Source: CAD feature listing. Evaluate the final solid. Frame: model axes, mm. Face numbers are marked on the shaded views. A direction names the side the tool comes from. Round coordinates to 2 decimals unless told otherwise and drop trailing zeros. Loops run counter-clockwise (first coordinate to the right, second up) from the corner with the lowest first, then second, coordinate; pieces in that order, holes last. Notation, with made-up numbers: M 48.5,-8 L 71.5,-8 A29 cw 71.5,20 Z; hole C 43,19.5 d1. An arc over 180 degrees is marked long. Answer as a JSON object with one key per item and string values.
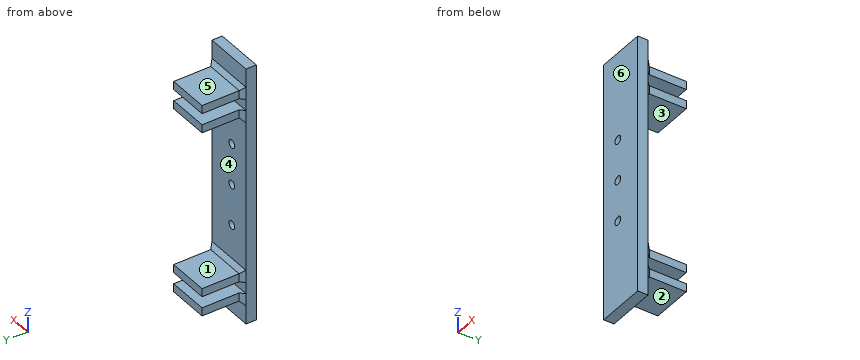
from build123d import *

# Parameters (mm, degrees)
SKETCH1_W               = 24
SKETCH1_H               = 126
BOSS_EXTRUDE1_DEPTH     = 5
SKETCH2_W               = 20
SKETCH2_H               = 4
BOSS_EXTRUDE2_DEPTH     = 20
CUT_EXTRUDE1_DEPTH      = 123.736336331
CUT_EXTRUDE1_DEPTH_BACK = 123.736336331
SKETCH3_R               = 2
CHAMFER1_SIZE           = 2


with BuildPart() as part:
    # Sketch1 → Boss-Extrude1 (new body)
    with BuildSketch(Plane(origin=(0, 0, 0), x_dir=(1, 0, 0), z_dir=(0, 1, 0))):
        with Locations((-62.650887574, -32.349112426)):
            Rectangle(SKETCH1_W, SKETCH1_H)
    extrude(amount=BOSS_EXTRUDE1_DEPTH)

    # Sketch2 → Boss-Extrude2 (add)
    with BuildSketch(Plane(origin=(0, 5, 0), x_dir=(1, 0, 0), z_dir=(0, 1, 0))):
        with Locations((-62.650887574, 17.650887574)):
            Rectangle(SKETCH2_W, SKETCH2_H)
        with Locations((-62.650887574, 8.150887574)):
            Rectangle(SKETCH2_W, SKETCH2_H)
        with Locations((-62.650887574, -72.849112426)):
            Rectangle(SKETCH2_W, SKETCH2_H)
        with Locations((-62.650887574, -82.349112426)):
            Rectangle(SKETCH2_W, SKETCH2_H)
    extrude(amount=BOSS_EXTRUDE2_DEPTH)

    # Sketch3 → Cut-Extrude1 (cut, two sides: drawn at the far end of the back side and taken through both)
    with BuildSketch(Plane(origin=(0, 5, 0), x_dir=(1, 0, 0), z_dir=(0, 1, 0)).offset(-CUT_EXTRUDE1_DEPTH_BACK)):
        with Locations(Location((-64.650887574, -32.349112426, 0), (0, 0, 270))):
            Circle(SKETCH3_R)
        with Locations(Location((-64.650887574, -12.349112426, 0), (0, 0, 270))):
            Circle(SKETCH3_R)
        with Locations(Location((-64.650887574, -52.349112426, 0), (0, 0, 270))):
            Circle(SKETCH3_R)
    extrude(amount=CUT_EXTRUDE1_DEPTH + CUT_EXTRUDE1_DEPTH_BACK, mode=Mode.SUBTRACT)

    # Chamfer1
    chamfer1_edges = [part.edges().sort_by_distance(p)[0] for p in [
        (-72.650887574, 5, -17.650887574),
        (-52.650887574, 5, -17.650887574),
        (-62.650887574, 5, -19.650887574),
        (-72.650887574, 5, -8.150887574),
        (-62.650887574, 5, -6.150887574),
        (-52.650887574, 5, -8.150887574),
        (-72.650887574, 5, 82.349112426),
        (-62.650887574, 5, 84.349112426),
        (-52.650887574, 5, 82.349112426),
        (-62.650887574, 5, 70.849112426),
        (-72.650887574, 5, 72.849112426),
        (-52.650887574, 5, 72.849112426),
    ]]
    chamfer(chamfer1_edges, length=CHAMFER1_SIZE - 0.0001)  # a hair under: the kernel refuses the full size


solid = part.part
Item 1: Access query for the marked faces 1 and 2. Directions: +Z, -Z, +X, -X, +Y, -Y. A direction counts if a zero-diameter tool reaches every point of the face in a straight line with its end or side. Return the directions, or none.
Answer sheet:
{"face 1": "+X, -X, +Y", "face 2": "-Z, +X, -X, +Y"}
Item 2: Section A-A on y = 11.75. Return the cut outline in (x, z), then the cut area to 3 significant figures.
Answer sheet:
{"outline": "M -72.65,-19.65 L -52.65,-19.65 L -52.65,-15.65 L -72.65,-15.65 Z; M -72.65,-10.15 L -52.65,-10.15 L -52.65,-6.15 L -72.65,-6.15 Z; M -72.65,70.85 L -52.65,70.85 L -52.65,74.85 L -72.65,74.85 Z; M -72.65,80.35 L -52.65,80.35 L -52.65,84.35 L -72.65,84.35 Z", "area": "320 mm²"}
Item 3: Section B-B on z = 53. Return the cut outline in (x, y), then the cut area to 3 significant figures.
Answer sheet:
{"outline": "M -74.65,0 L -66.54,0 L -66.54,5 L -74.65,5 Z; M -62.76,0 L -50.65,0 L -50.65,5 L -62.76,5 Z", "area": "101 mm²"}
Item 4: Section C-C on x = -69.5. Return the cut outline in (y, z).
Answer sheet:
{"outline": "M 0,-30.65 L 5,-30.65 L 5,-21.65 L 7,-19.65 L 25,-19.65 L 25,-15.65 L 5,-15.65 L 5,-10.15 L 25,-10.15 L 25,-6.15 L 7,-6.15 L 5,-4.15 L 5,68.85 L 7,70.85 L 25,70.85 L 25,74.85 L 5,74.85 L 5,80.35 L 25,80.35 L 25,84.35 L 7,84.35 L 5,86.35 L 5,95.35 L 0,95.35 Z"}
Item 5: Contact query for flat-ended pins moving along their axis: pin 1 Ø1 at (x, z) = (-55, 40.5) entering from +Y; pin 2 Ø8 at (y, z) = (19, 72.5) entering from -X; pin 3 Ø10 at (x, y) = (-69, 13) entering from +Z. Output: stop coordinate, or through.
Answer sheet:
{"pin 1": "stops at y = 5", "pin 2": "stops at x = -72.65", "pin 3": "stops at z = 84.35"}
Item 6: Line query: probe 1 along Z at (x, y) = (-69.5, 16.25); probe 2 along Z at (x, y) = (-55.75, 6.75); probe 3 along Y at (x, z) = (-56.25, 39.5). Output: solid intervals per line, ascending. Write a range as from..to.
Answer sheet:
{"probe 1": "z = -19.65..-15.65, -10.15..-6.15, 70.85..74.85, 80.35..84.35", "probe 2": "z = -19.9..-15.65, -10.15..-5.9, 70.6..74.85, 80.35..84.6", "probe 3": "y = 0..5"}
Item 7: Pull-direction query (Z, two-part tool) for the marked faces 3, 4, 5 and 6; classes: pulls with the +Z half, pulls with the -Z half, needs draft (parallel to the pull), parting line crosses it, or undercut.
Answer sheet:
{"face 3": "undercut", "face 4": "undercut", "face 5": "pulls with the +Z half", "face 6": "needs draft"}
